Autodesk Inventor part; units mm, degrees
ref_plane "Work Plane3" through (0, 0, 5) normal (0, 0, 1) x (1, 0, 0)
ref_plane "Work Plane4" through (0, 0, 28) normal (0, 0, 1) x (1, 0, 0)
ref_plane "YZ Plane" through (0, 0, 0) normal (1, 0, 0) x (0, 1, 0)
sketch "Sketch1" plane through (0, 0, 0) normal (0, 0, 1) x (1, 0, 0)
  circle A0 centre (0, 0) radius 0.3405
  dimension "d0" = 0.681
ref_plane "Work Plane1" through (0, 0, 1) normal (0, 0, 1) x (1, 0, 0)
sketch "Sketch2" plane through (0, 0, 1) normal (0, 0, 1) x (1, 0, 0)
  circle A0 centre (0, 0) radius 1.0215
  dimension "d2" = 2.043
ref_plane "Work Plane2" through (0, 0, 4) normal (0, 0, 1) x (1, 0, 0)
sketch "Sketch3" plane through (0, 0, 4) normal (0, 0, 1) x (1, 0, 0)
  circle A0 centre (0, 0) radius 0.8476
  dimension "d4" = 1.6951
ref_plane "Work Plane3" through (0, 0, 5) normal (0, 0, 1) x (1, 0, 0)
sketch "Sketch4" plane through (0, 0, 5) normal (0, 0, 1) x (1, 0, 0)
  circle A0 centre (0, 0) radius 1.1935
  dimension "d6" = 2.387
loft "Loft1" add profiles "Sketch4", "Sketch3"
loft "Loft2" add profiles "Sketch2" section 1 edges at (-0.8476, 0, 4)
loft "Loft3" add profiles "Sketch1" section 2 edges at (-1.0215, 0, 1)
sketch "Sketch5" plane through (0, 0, 5) normal (0, 0, 1) x (1, 0, 0)
  circle A0 centre (0, 0) radius 1.1906
  dimension "d35" = 2.3813
extrude "Extrusion1" add sketch "Sketch5" along normal blind 10
sketch "Sketch6" plane through (0, 0, 15) normal (0, 0, 1) x (1, 0, 0)
  circle A0 centre (0, 0) radius 1.7038
  dimension "d21" = 3.4076
extrude "Extrusion2" add sketch "Sketch6" along normal blind 10
ref_plane "Work Plane4" through (0, 0, 28) normal (0, 0, 1) x (1, 0, 0)
sketch "Sketch7" plane through (0, 0, 28) normal (0, 0, 1) x (1, 0, 0)
  arc A0 (-0.635, 0.635) -> (-0.635, -0.635) centre (-0.635, 0) ccw
  arc A1 (0.635, -0.635) -> (0.635, 0.635) centre (0.635, 0) ccw
  line L0 (-0.635, 0.635) -> (0.635, 0.635)
  line L1 (0.635, -0.635) -> (-0.635, -0.635)
loft "Loft4" add profiles "Sketch7" section 1 edges at (-1.7038, 0, 25)
sketch "Sketch8" plane through (0, 0, 28) normal (0, 0, 1) x (1, 0, 0)
  arc A0 (-0.635, 0.635) -> (-0.635, -0.635) centre (-0.635, 0) ccw
  circle A1 centre (-0.635, 0) radius 0.635
  arc A2 (0.635, -0.635) -> (0.635, 0.635) centre (0.635, 0) ccw
  circle A3 centre (0.635, 0) radius 0.635
  point P0 (0, 0)
extrude "Extrusion3" add sketch "Sketch8" along normal blind 25.4
properties part number "Male End Audio Jack"
Design review of the part built by this model. Coordinates are the model's own, in mm. A direction names the side the tool comes from. Round coordinates to 2 decimals unless told otherwise and drop trailing zeros.
Item 1: Draft analysis for pull direction Z (two halves, no side actions). For faces 4 (the conical face through (-0.203, 0.914, 2.479)), 5 (the flat face through (1, -1, 15)), 6 (the flat face through (1, 0, 53.4)), state which applies: released by +Z, released by -Z, zero draft, split by the parting line, or undercut.
Item 2: For pin 1 Ø1 at (y, z) = (0.5, 44.5) entering from +X; pin 2 Ø1.5 at (x, z) = (0, 32) entering from +Y (3 decimals); pin 3 Ø1 at (y, z) = (0.5, 13.5) entering from +X, all flat-tipped, find the tip position at first contact; note any pin that passes through.
Item 3: Wall thickness on L1, parallel to X at y = -0.1, z = 23; L2, parallel to Y at x = -1, z = 6.5; L3, parallel to X at y = 0.1, z = 12: over which ranges is each line inside the solid? List them lowest first.
Item 4: For faces 1 (the cylindrical face through (-0.26, 1.16, 9.93)), 2 (the conical face through (-0.197, -0.886, 4.174)), 3 (the flat face through (-1, 0, 53.4)), list the 3-axis set-ups (+Z, -Z, +X, -X, +Y, -Y) from which the entire face can be reached by the end or side of a thin tool; tool diameter is ignored.
Check values:
1. face 4: undercut
1. face 5: released by -Z
1. face 6: released by +Z
2. pin 1: stops at x = 1.27
2. pin 2: stops at y = 0.635
2. pin 3: stops at x = 1.19
3. L1: x = -1.7 to 1.7
3. L2: y = -0.65 to 0.65
3. L3: x = -1.19 to 1.19
4. face 1: -Z
4. face 2: none
4. face 3: +Z, +X, -X, +Y, -Y
